Check sheet for the modelled part. Datum: model origin and axes. Units: mm. A direction names the side the tool comes from. Give positions to 0.01 mm unless a question says otherwise; leave off trailing zeros. Loops run counter-clockwise (first coordinate to the right, second up) from the corner with the lowest first, then second, coordinate; pieces in that order, holes last. Notation, with made-up numbers: (-25, 49) - (-17, 49) arc R35 cw to (-17, 86) - close; hole circle Ø1 at (82.25, 52.5). An arc over 180 degrees is marked (long way). Answer in a Markdown table with one row per item. Add a question column.
(1) Sectioned sample at A-A on x = 0. Enter the section's corners in (y, z), then the cut area to 3 significant figures.
(2) Sectioned sample at C-C on z = 4.25. Enter the section's corners in (x, y), then the cut area to 3 significant figures.
(3) Thickness scan on L1, parallel to X at y = 0, z = 2.2; L2, parallel to X at y = 0, z = 7.75. Record the ranges inside material, lowest first.
(4) Go/stop test with flat-tipped pins: P1, Ø2, axis at y = 0, z = 6.5, coming from the +X side; P2, Ø2, axis at y = 1.5, z = 11, coming from the -X side. Record where each tip stops, or that it passes through.
(5) Draft check along X on faces 3 (the face through (1, -3, 1.2)), 4 (the face through (-0.631, -2.003, 8.623)), 5 (the face through (0.585, -2.636, 7.412)). Enter one of: released by +X, released by -X, zero draft, split by the parting line, or undercut.
(6) Set-up check for faces 1 (the face through (-0.66, 2.1, 1.62)), 2 (the face through (-2, -2, 0)): record each of +Z, -Z, +X, -X, +Y, -Y from which the full face is reachable in a straight line by a thin tool's end or side.
Autodesk Fusion 360 part; units mm, degrees
sketch "Sketch1" plane through (0, 0, 0) normal (0, 0, 1) x (1, 0, 0)
  circle A0 centre (0, 0) radius 3.5
  dimension "d1" = 7
extrude "Extrude1" add sketch "Sketch1" along normal blind 1.2
sketch "Sketch2" plane through (0, 0, 1.2) normal (0, 0, 1) x (-1, 0, 0)
  circle A0 centre (0, 0) radius 3.5
  circle A1 centre (0, 0) radius 2.7
  dimension "d4" = 5.4
extrude "Extrude2" add sketch "Sketch2" along normal blind 13 contours A1
chamfer "Chamfer1" distance 0.4 angle 45 1 edges at (2.5173, 0.9764, 14.2)
sketch "Sketch3" plane through (0, 0, 14.2) normal (0, 0, 1) x (-1, 0, 0)
  circle A0 centre (0, 0) radius 2.3
  circle A1 centre (0, 0) radius 1.9
  dimension "d8" = 3.8
hole "Hole1" at (0, 0, 14.2) direction (0, 0, -1) diameter 4.2 depth 11 tip angle 180
sketch "Sketch4" plane through (0, 0, 0) normal (0, 0, -1) x (1, 0, 0)
  circle A0 centre (0, 0) radius 3.5
  circle A1 centre (0, 0) radius 2.2
  dimension "d12" = 4.4
hole "Hole2" at (0, 0, 0) direction (0, 0, 1) diameter 4.4 depth 3.2 tip angle 180
Reply:
| question | item | result |
|---|---|---|
| 1 | outline | (-3.5, 0) - (-2.2, 0) - (-2.2, 3.2) - (-2.1, 3.2) - (-2.1, 14.2) - (-2.3, 14.2) - (-2.7, 13.8) - (-2.7, 1.2) - (-3.5, 1.2) - close; (2.1, 3.2) - (2.2, 3.2) - (2.2, 0) - (3.5, 0) - (3.5, 1.2) - (2.7, 1.2) - (2.7, 13.8) - (2.3, 14.2) - (2.1, 14.2) - close |
| 1 | area | 18.2 mm^2 |
| 2 | outline | circle Ø5.4 at (0, 0); hole circle Ø4.2 at (0, 0) |
| 2 | area | 9.05 mm^2 |
| 3 | L1 | -2.7 to -2.2, 2.2 to 2.7 |
| 3 | L2 | -2.7 to -2.1, 2.1 to 2.7 |
| 4 | P1 | x = 2.7 |
| 4 | P2 | x = -2.65 |
| 5 | face 3 | zero draft |
| 5 | face 4 | undercut |
| 5 | face 5 | split by the parting line |
| 6 | face 1 | -Z |
| 6 | face 2 | -Z, +X, -X, +Y, -Y |
